Geometry: see drawing. Coordinates: mm, zero at the bounding-box minimum. A direction names the side the tool comes from. Give positions to 0.01 mm unless a question says otherwise; leave off trailing zeros. Answer as a JSON object with one key per item and string values. Group by question number.
1. Material intervals for L1, parallel to Z at x = 1, y = 2.5; L2, parallel to Y at x = 4.75, z = 7.75 (1 decimal); L3, parallel to Y at x = 3.75, z = 4.25 (1 decimal), sorted ascending. Write a range as [from, to].
2. Set-up query: the marked faces 1, 2 and 3. Return all of +Z, -Z, +X, -X, +Y, -Y with unobstructed straight access to the full face (end or side cutting, diameter ignored); none if empty.
3. Pin query (flat end, axial travel): P1, Ø1.5, axis at x = 6, z = 1.5, coming from the +Y side (1 decimal). Return the tip coordinate at first contact, or that it passes through.
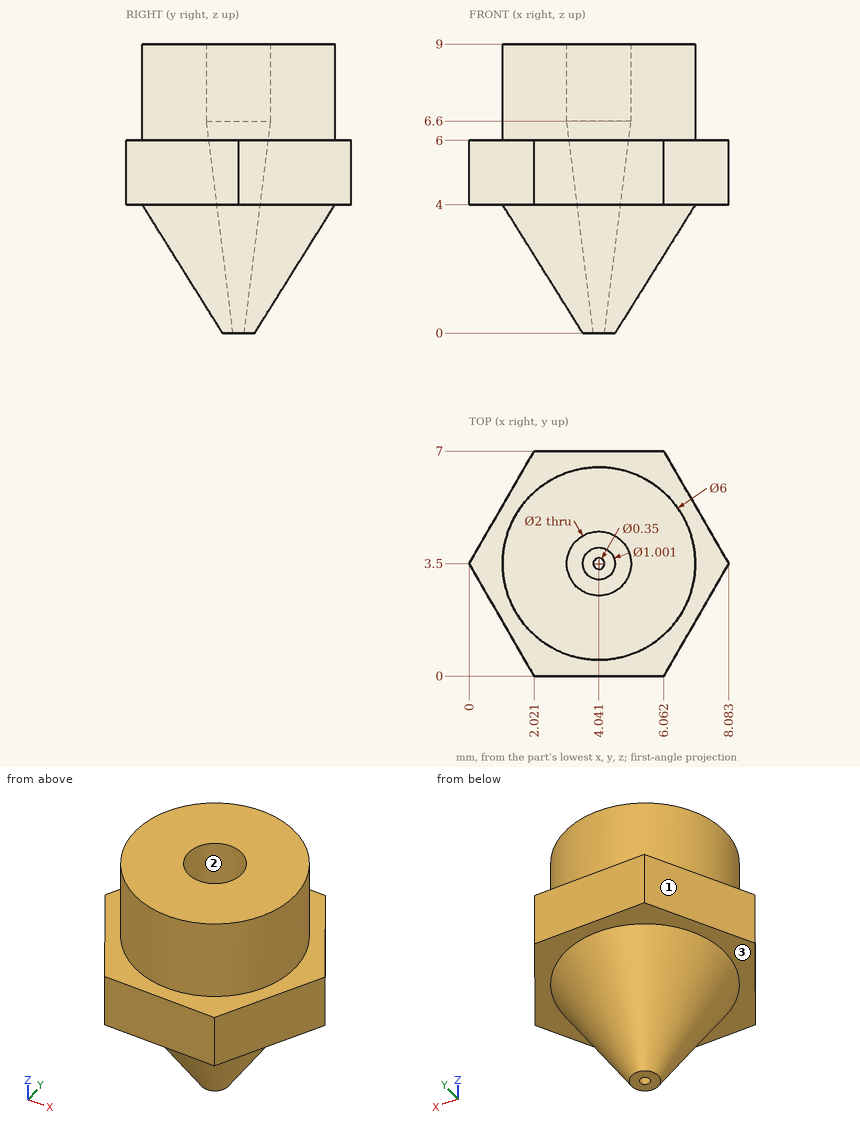
Answer sheet:
{
 "1": {"L1": "[4, 6]", "L2": "[0.6, 2.8], [4.2, 6.4]", "L3": "[0, 2.9], [4.1, 7]"},
 "2": {"face 1": "+Z, -Z, -X, +Y", "face 2": "+Z", "face 3": "-Z"},
 "3": {"P1": "y = 4.6"}
}
